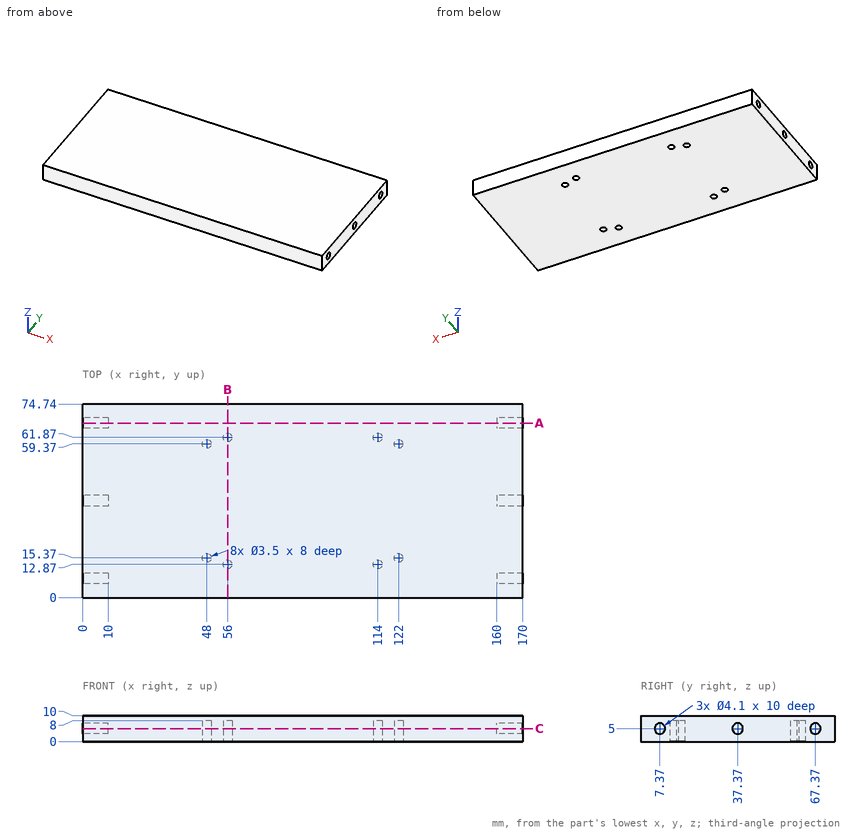
Geometry check sheet. Reference: drawing and pictorial views, mm from the part's lowest x, y, z. Coordinates: 2 decimals unless noted, no trailing zeros. Order: outer loops, then holes, each group sorted by start corner. A loop starts at its lowest first (then second) coordinate and runs counter-clockwise, first axis right, second up.
Item 1: Depth check by flat-ended pin: pin 1 (1.8 mm diameter, centred on x = 121.5, y = 15.5, fed in from -Z); pin 2 (2.5 mm diameter, centred on y = 7.37, z = 5, fed in from +X). Enter the tip coordinate at first touch or a pass-through.
Item 2: Section check B-B (x = 56). Enter the section's corners in (y, z), plus the area to 3 significant figures.
Item 3: Section check A-A (y = 67.37). Enter the section's corners in (x, z), plus the area to 3 significant figures.
Item 4: Scan lines: line 1 along Y through (x, z) = (163.5, 5); line 2 along Y through (x, z) = (122, 5.5); line 3 along X through (y, z) = (15.37, 3.5). Record each from-to range of solid material in increasing order.
Item 5: Section check C-C (z = 5). Count the separate pieces of the cut face and the enclosed holes in it, plus the area to 3 significant figures.
Check sheet entries:
1. pin 1: stops at z = 8
1. pin 2: stops at x = 160
2. outline: (0, 0) - (11.12, 0) - (11.12, 8) - (14.62, 8) - (14.62, 0) - (60.12, 0) - (60.12, 8) - (63.62, 8) - (63.62, 0) - (74.74, 0) - (74.74, 10) - (0, 10) - close
2. area: 691 mm2
3. outline: (0, 0) - (170, 0) - (170, 2.95) - (160, 2.95) - (160, 7.05) - (170, 7.05) - (170, 10) - (0, 10) - (0, 7.05) - (10, 7.05) - (10, 2.95) - (0, 2.95) - close
3. area: 1,620 mm2
4. line 1: y = 0 to 5.32, 9.42 to 35.32, 39.42 to 65.32, 69.42 to 74.74
4. line 2: y = 0 to 13.62, 17.12 to 57.62, 61.12 to 74.74
4. line 3: x = 0 to 46.25, 49.75 to 120.25, 123.75 to 170
5. separate pieces: 1
5. enclosed holes: 8
5. area: 12,400 mm2
